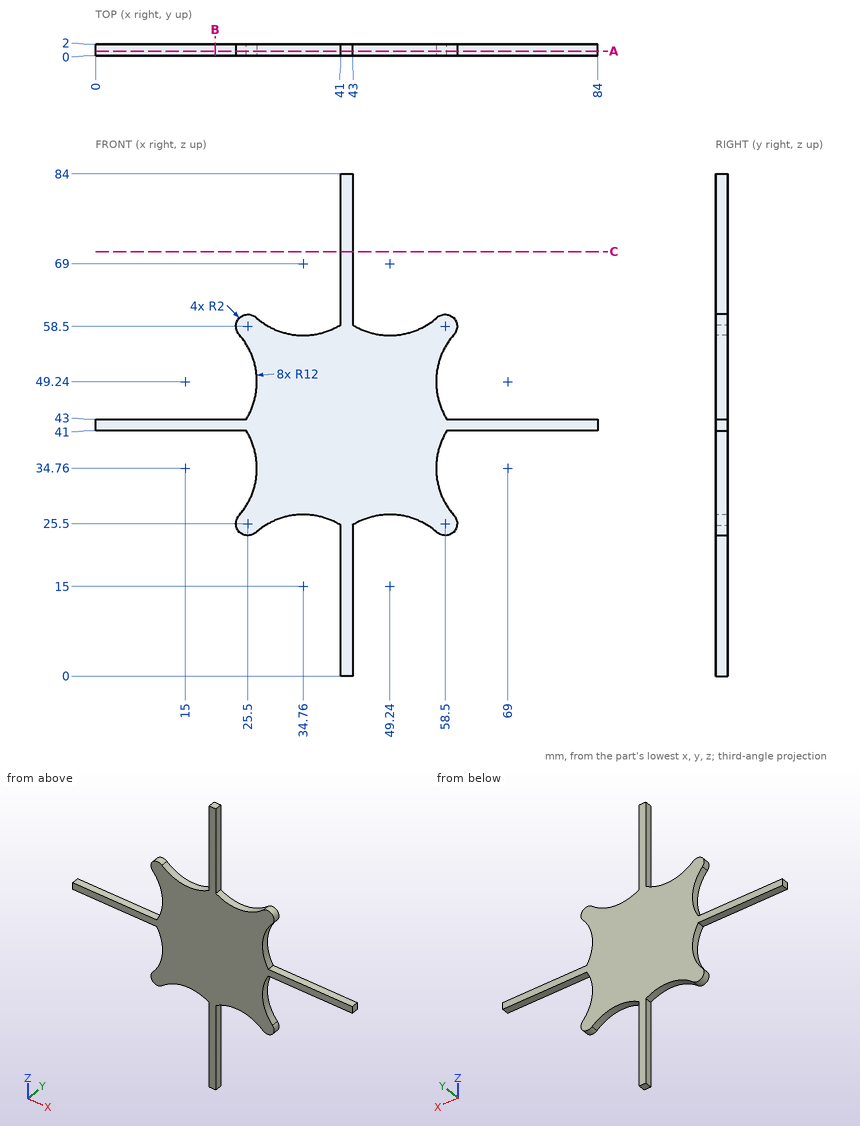
Input: dimensioned drawing with shaded views. Units: mm. Origin: part minimum x, y, z. Round coordinates to 2 decimals unless told otherwise and drop trailing zeros. Loops run counter-clockwise (first coordinate to the right, second up) from the corner with the lowest first, then second, coordinate; pieces in that order, holes last. Notation, with made-up numbers: M 76,64.25 L 127,64.25 A21 ccw 127,72.25 Z; hole C -37,24.5 d10. An arc over 180 degrees is marked long. Answer in a Markdown table with one row per item. Add a question column.
1. Section A-A (y = 0.8). Output: boundary loops of the cut face in (x, z), and give its area (3 significant figures).
2. Section B-B (x = 20). Output: boundary loops of the cut face in (y, z).
3. Ray query, probe 1 along X at (y, z) = (0.1, 25); probe 2 along X at (y, z) = (1.7, 80); probe 3 along Z at (x, y) = (25.5, 1.7). Return the intervals inside material, ascending.
4. Section C-C (z = 71). Output: boundary loops of the cut face in (x, y).
5. Contact query for flat-ended pins moving along their axis: pin 1 (1 mm diameter, centred on y = 0.5, z = 75.5, fed in from -X); pin 2 (0.6 mm diameter, centred on x = 7, y = 1.5, fed in from +Z); pin 3 (1 mm diameter, centred on x = 27, y = 0.5, fed in from +Z). Output: stop coordinate, or through.
Values follow:
| question | item | result |
|---|---|---|
| 1 | outline | M 0,41 L 25.25,41 A12 cw 24,26.82 A2 ccw 26.82,24 A12 cw 41,25.25 L 41,0 L 43,0 L 43,25.25 A12 cw 57.18,24 A2 ccw 60,26.82 A12 cw 58.75,41 L 84,41 L 84,43 L 58.75,43 A12 cw 60,57.18 A2 ccw 57.18,60 A12 cw 43,58.75 L 43,84 L 41,84 L 41,58.75 A12 cw 26.82,60 A2 ccw 24,57.18 A12 cw 25.25,43 L 0,43 Z |
| 1 | area | 1,240 mm^2 |
| 2 | outline | M 0,41 L 2,41 L 2,43 L 0,43 Z |
| 3 | probe 1 | 23.56 to 28.13, 41 to 43, 55.87 to 60.44 |
| 3 | probe 2 | 41 to 43 |
| 3 | probe 3 | 23.5 to 28.95, 40.57 to 43.43, 55.05 to 60.5 |
| 4 | outline | M 41,0 L 43,0 L 43,2 L 41,2 Z |
| 5 | pin 1 | x = 41 |
| 5 | pin 2 | z = 43 |
| 5 | pin 3 | z = 60.23 |
